```python
from build123d import *

# Parameters (mm, degrees)
F5_R     = 20
F6_DEPTH = 5


with BuildPart() as f1:
    # F0 (on Front) → F1 (revolve)
    with BuildSketch(Plane.XZ):
        with BuildLine():
            Line((-6.8241658505, -19.05), (-4.9969541351, -71.3744974835))
            ThreePointArc((-4.9969541351, -71.3744974835), (-3.4732918523, -74.7966990017), (0, -76.2))
            Line((0, -76.2), (0, 0))
            Line((0, 0), (0, 20))
            Line((0, 20), (-7.8225340458, 20))
            Line((-7.8225340458, 20), (-7.8225340458, 0))
            Line((-7.8225340458, 0), (-6.8241658505, -19.05))
        make_face()
    revolve(axis=Axis((0, 0, 4.3368881511), (0, 0, -1)))

    # F3 (on Front) → F4 (revolve)
    with BuildSketch(Plane.XZ):
        Polygon((9.9000765866, 21.2795146775), (-5, 0), (27.5109955121, 2.8443435472), (30.3788776938, 6.9401037687), align=None)
    revolve(axis=Axis((2.4500382933, 0, 10.6397573387), (0.5735764364, 0, 0.8191520443)))

    # F5 (on face) → F6 (cut)
    with BuildSketch(Plane(origin=(13.2551269449, 0, 18.9302831255), x_dir=(0.8191520443, 0, -0.5735764364), z_dir=(0.5735764364, 0, 0.8191520443))):
        with Locations((-4.0957602214, 0)):
            Circle(F5_R)
    extrude(amount=-F6_DEPTH, mode=Mode.SUBTRACT)


solid = f1.part
```
The listing builds one solid part. Answer for the finished solid, in the listing's coordinates (mm). A direction names the side the tool comes from. Round coordinates to 2 decimals unless told otherwise and drop trailing zeros. Loops run counter-clockwise (first coordinate to the right, second up) from the corner with the lowest first, then second, coordinate; pieces in that order, holes last. Notation, with made-up numbers: (29, 21) - (45, 21) arc R31 ccw to (45, 56) - close; hole circle Ø1 at (46, 61). An arc over 180 degrees is marked (long way). Use one line per item in the form item = value. Start each with the question number.
1. Given pin 1 Ø3 at (x, z) = (-0.5, -50) entering from -Y; pin 2 Ø1 at (x, y) = (7.5, 17) entering from -Z; pin 3 Ø4 at (x, z) = (18.5, 14) entering from +Y, each flat-ended and moving along its own axis, determine where each tip first touches the part or whether it passes through.
2. Consider line 1 (Z direction, x = 0, y = 15); line 2 (Z direction, x = 22, y = 19.5); line 3 (X direction, y = -4, z = -66). Determine where each line is inside the solid, lowest interval first. Write a range as [from, to].
3. A tool of negligible diameter and unlimited length cuts with its end or side. For faces 4 (the face through (4.935, -19.524, 21.747)), 5 (the face through (1.279, -5.758, -45.579)), from which of +Z, -Z, +X, -X, +Y, -Y can it reach the whole face along a straight path? Write none if from no direction.
4. For a pull along X with two mould halves and no side action, classify faces 1 (the face through (0.7, 16.78, 27.72)), 2 (the face through (6.803, 0.28, 17.344)), 3 (the face through (1.59, -7.14, -9.66)) as pulls with the +X half, pulls with the -X half, needs draft (parallel to the pull), parting line crosses it, or undercut.
5. The part is cut by section A-A on y = 0. Determine the outline of the cut face in (x, z), then the cut area to 3 significant figures.
6. The part is cut by section B-B on z = -6.5. Determine the outline of the cut face in (x, y).
Geometry check:
q1.pin_1 = -5.79
q1.pin_2 = 8.9
q1.pin_3 = 23.24
q2.line_1 = [12.14, 22.11]
q2.line_2 = [11.28, 12.81]
q2.line_3 = [-3.3, 3.3]
q3.face_4 = none
q3.face_5 = -Z
q4.face_1 = pulls with the +X half
q4.face_2 = undercut
q4.face_3 = parting line crosses it
q5.outline = (-13.45, 31.52) - (-7.82, 10.53) - (-7.82, 0) - (-6.82, -19.05) - (-5, -71.37) arc R5 ccw to (5, -71.37) - (6.82, -19.05) - (7.82, 0) - (7.82, 1.12) - (27.51, 2.84) - (30.38, 6.94) - (26.28, 9.81) - (23.42, 5.71) - (-9.35, 28.66) - (-6.48, 32.75) - (-10.58, 35.62) - close
q5.area = 1,530 mm^2
q6.outline = circle Ø14.96 at (0, 0)
